Autodesk Inventor part; units mm, degrees
ref_plane "YZ Plane" through (0, 0, 0) normal (1, 0, 0) x (0, 1, 0)
ref_plane "XZ Plane" through (0, 0, 0) normal (0, 1, 0) x (-1, 0, 0)
ref_plane "XY Plane" through (0, 0, 0) normal (0, 0, 1) x (1, 0, 0)
sketch "Boceto1" plane through (0, 0, 0) normal (0, 0, 1) x (1, 0, 0)
  circle A0 centre (690.2291, 250.8095) radius 1.25
  arc A1 (692.4377, 251.981) -> (691.1952, 248.5037) centre (690.2291, 250.8095) ccw
  circle A2 centre (705.5291, 233.3595) radius 1.25
  line L0 (692.5597, 251.7803) -> (703.1648, 236.452)
  line L1 (692.3398, 247.8801) -> (702.5235, 233.1607)
  arc A3 (702.665, 232.951) -> (702.6433, 232.9876) centre (702.3966, 232.8169) ccw
  arc A4 (703.9859, 231.7221) -> (705.2332, 235.59) centre (705.5291, 233.3595) ccw
  line L2 (702.7965, 232.8432) -> (703.9859, 231.7221)
  line L3 (704.8095, 235.59) -> (705.2332, 235.59)
  arc A5 (703.1648, 236.452) -> (704.8095, 235.59) centre (704.8095, 237.59) ccw
  arc A6 (702.5235, 233.1607) -> (702.7965, 232.8432) centre (704.1683, 234.2986) ccw
  line L4 (692.3398, 247.8801) -> (691.1952, 248.5037)
  arc A7 (692.4377, 251.981) -> (692.5597, 251.7803) centre (694.2045, 252.9182) ccw
  point P0 (0, 0)
  dimension "d7" = 2.5
  dimension "d8" = 5
  dimension "d9" = 2.5
  dimension "d11" = 15.3
  dimension "d12" = 17.45
  dimension "d18" = 4.5
  dimension "d19" = 2
  dimension "d20" = 2.4
  dimension "d21" = 2
extrude "Extrusión1" add sketch "Boceto1" along normal blind 1.2
properties part number "Pieza9_3DPrint"
Check sheet for the modelled part. Datum: model origin and axes. Units: mm. A direction names the side the tool comes from. Coordinates: 2 decimals unless noted, no trailing zeros. Write each loop counter-clockwise with the first axis right and the second up, starting at its lowest first coordinate (ties: lowest second). Pieces come first, ordered by that corner, then holes.
Item 1: Cross-section at A-A on x = 690.75. Record the boundary of the cut face in (y, z).
Numbers:
outline: (248.36, 0) - (249.67, 0) - (249.67, 1.2) - (248.36, 1.2) - close; (251.95, 0) - (253.25, 0) - (253.25, 1.2) - (251.95, 1.2) - close
Item 2: Cross-section at B-B on z = 0.95. Record the boundary of the cut face in (x, y), then the cut area to 3 significant figures.
Numbers:
outline: (691.2, 248.5) - (692.34, 247.88) - (702.52, 233.16) arc R2 ccw to (702.8, 232.84) - (703.99, 231.72) arc R2.25 ccw (long way) to (705.23, 235.59) - (704.81, 235.59) arc R2 cw to (703.16, 236.45) - (692.56, 251.78) arc R2.02 cw to (692.44, 251.98) arc R2.5 ccw (long way) to start; hole circle Ø2.5 at (690.23, 250.81); hole circle Ø2.5 at (705.53, 233.36)
area: 73.4 mm2
Item 3: Scan lines: probe 1 along Y at (x, z) = (705.5, 0.6); probe 2 along X at (y, z) = (233.5, 0.9); probe 3 along Y at (x, z) = (690.5, 0.45). Record each from-to range of solid material in increasing order.
Numbers:
probe 1: y = 231.11 to 232.11, 234.61 to 235.61
probe 2: x = 702.29 to 704.29, 706.77 to 707.77
probe 3: y = 248.32 to 249.59, 252.03 to 253.29
Item 4: Cross-section at C-C on x = 705.5. Record the boundary of the cut face in (y, z), then the cut area to 3 significant figures.
Numbers:
outline: (231.11, 0) - (232.11, 0) - (232.11, 1.2) - (231.11, 1.2) - close; (234.61, 0) - (235.61, 0) - (235.61, 1.2) - (234.61, 1.2) - close
area: 2.40 mm2
Item 5: Access from +Z, -Z, +X, -X, +Y, -Y to the whole of each face (thin tool, end or side, straight path). Record for faces 1 (the face through (691.776, 248.188, 0.592)), 2 (the face through (703.383, 232.29, 0.592)).
Numbers:
face 1: +Z, -Z, -Y
face 2: +Z, -Z, -X, -Y
Item 6: Depth check by flat-ended pin: pin 1 Ø6 at (x, y) = (697, 234) entering from +Z. Enter the tip coordinate at first touch or a pass-through.
Numbers:
pin 1: passes through
Item 7: Mould release check, pull along X, two halves, no side actions. Record for faces 3 (the face through (697.36, 240.623, 0.592)), 4 (the face through (691.42, 250.43, 0.59)), 5 (the face through (698, 242, 1.2)): released by +X, released by -X, zero draft, split by the parting line, or undercut.
Numbers:
face 3: released by -X
face 4: undercut
face 5: zero draft
Item 8: Cross-section at D-D on y = 246. Record the boundary of the cut face in (x, z), then the cut area to 3 significant figures.
Numbers:
outline: (693.64, 0) - (696.56, 0) - (696.56, 1.2) - (693.64, 1.2) - close
area: 3.50 mm2
